```python
from build123d import *
from build123d.topology import SkipClean

# Parameters (mm, degrees)
SKETCH1_R           = 8.75
SKETCH1_R_2         = 4.25
SKETCH1_R_3         = 1.25
BOSS_EXTRUDE1_DEPTH = 1.8
SKETCH2_R           = 2
CUT_EXTRUDE1_DEPTH  = 0.6
SKETCH3_R           = 1.45
BOSS_EXTRUDE2_DEPTH = 1.5
FILLET1_R           = 5
CHAMFER1_SIZE       = 0.7
CHAMFER2_SIZE       = 0.7


with BuildPart() as part:
    # Sketch1 → Boss-Extrude1 (new body)
    with BuildSketch(Plane(origin=(0, 0, 0), x_dir=(1, 0, 0), z_dir=(0, 1, 0))):
        with Locations(Location((0, 0, 0), (0, 0, 270))):
            Circle(SKETCH1_R)
        with Locations(Location((0, 0, 0), (0, 0, 270))):
            Circle(SKETCH1_R_2, mode=Mode.SUBTRACT)
        with Locations(Location((-6, 0, 0), (0, 0, 270))):
            Circle(SKETCH1_R_3, mode=Mode.SUBTRACT)
        with Locations(Location((6, 0, 0), (0, 0, 270))):
            Circle(SKETCH1_R_3, mode=Mode.SUBTRACT)
    extrude(amount=BOSS_EXTRUDE1_DEPTH)

    # Sketch2 → Cut-Extrude1 (cut)
    with BuildSketch(Plane(origin=(0, 1.8, 0), x_dir=(1, 0, 0), z_dir=(0, 1, 0))):
        with Locations((-6, 0)):
            Circle(SKETCH2_R)
        with Locations((6, 0)):
            Circle(SKETCH2_R)
    extrude(amount=-CUT_EXTRUDE1_DEPTH, mode=Mode.SUBTRACT)

    # Sketch3 → Boss-Extrude2 (add)
    with SkipClean():  # the faces are left unmerged after this step: merging them gives an invalid solid
        with BuildSketch(Plane.XZ.offset(-1.8)):
            with BuildLine():
                Line((-22.592922776, -20.580461491), (-13.466151705, -20.580461491))
                ThreePointArc((-13.466151705, -20.580461491), (0, -11.838443279), (13.466151705, -20.580461491))
                Line((13.466151705, -20.580461491), (22.592922776, -20.580461491))
                Line((22.592922776, -20.580461491), (22.592922776, -12.644988276))
                ThreePointArc((22.592922776, -12.644988276), (15.601572689, 0), (22.592922776, 12.644988276))
                Line((22.592922776, 12.644988276), (22.592922776, 20.580461491))
                Line((22.592922776, 20.580461491), (13.466151705, 20.580461491))
                ThreePointArc((13.466151705, 20.580461491), (0, 11.838443279), (-13.466151705, 20.580461491))
                Line((-13.466151705, 20.580461491), (-22.592922776, 20.580461491))
                Line((-22.592922776, 20.580461491), (-22.592922776, 12.644988276))
                ThreePointArc((-22.592922776, 12.644988276), (-15.601572689, 0), (-22.592922776, -12.644988276))
                Line((-22.592922776, -12.644988276), (-22.592922776, -20.580461491))
            make_face()
            with Locations(Location((18.75, 16.75, 0), (0, 0, 270))):
                Circle(SKETCH3_R, mode=Mode.SUBTRACT)
            with Locations(Location((18.75, -16.75, 0), (0, 0, 270))):
                Circle(SKETCH3_R, mode=Mode.SUBTRACT)
            with Locations(Location((-18.75, -16.75, 0), (0, 0, 270))):
                Circle(SKETCH3_R, mode=Mode.SUBTRACT)
            with Locations(Location((-18.75, 16.75, 0), (0, 0, 270))):
                Circle(SKETCH3_R, mode=Mode.SUBTRACT)
            with BuildLine():
                ThreePointArc((-4.171875, -0.81114671), (0, -4.25), (4.171875, -0.81114671))
                ThreePointArc((4.171875, -0.81114671), (8, 0), (4.171875, 0.81114671))
                ThreePointArc((4.171875, 0.81114671), (0, 4.25), (-4.171875, 0.81114671))
                ThreePointArc((-4.171875, 0.81114671), (-8, 0), (-4.171875, -0.81114671))
            make_face(mode=Mode.SUBTRACT)
        extrude(amount=-BOSS_EXTRUDE2_DEPTH)

    # Fillet1
    fillet1_edges = [part.edges().sort_by_distance(p)[0] for p in [
        (13.466151705, 2.55, 20.580461491),
        (22.592922776, 2.55, 20.580461491),
        (22.592922776, 2.55, 12.644988276),
        (22.592922776, 2.55, -12.644988276),
        (22.592922776, 2.55, -20.580461491),
        (13.466151705, 2.55, -20.580461491),
        (-13.466151705, 2.55, -20.580461491),
        (-22.592922776, 2.55, -20.580461491),
        (-22.592922776, 2.55, -12.644988276),
        (-22.592922776, 2.55, 12.644988276),
        (-22.592922776, 2.55, 20.580461491),
        (-13.466151705, 2.55, 20.580461491),
    ]]
    fillet(fillet1_edges, radius=FILLET1_R)

    # Chamfer1
    # the kernel refuses this chamfer: 0.7 mm, written as the material it takes off along each edge
    with BuildSketch(Plane(origin=(0, 0, 0), x_dir=(0, 0, 1), z_dir=(-1, 0, 0))) as chamfer1_piece_1:
        Polygon((8.75, CHAMFER1_SIZE), (8.75 - CHAMFER1_SIZE, 0), (8.75, 0), align=None)
    revolve(axis=Axis((0, 0, 0), (0, 1, 0)), mode=Mode.SUBTRACT)
    with BuildSketch(Plane(origin=(0, 0, 0), x_dir=(0, 0, 1), z_dir=(-1, 0, 0))) as chamfer1_piece_2:
        Polygon((4.25 + CHAMFER1_SIZE, 0), (4.25, CHAMFER1_SIZE), (4.25, 0), align=None)
    revolve(axis=Axis((0, 0, 0), (0, 1, 0)), mode=Mode.SUBTRACT)

    # Chamfer2
    chamfer2_edges = [part.edges().sort_by_distance(p)[0] for p in [
        (15.601572689, 3.3, 0),
        (16.993372755, 3.3, 20.580461491),
        (22.592922776, 3.3, 15.369960777),
        (16.993372755, 3.3, -20.580461491),
        (0, 3.3, -11.838443279),
        (-16.993372755, 3.3, -20.580461491),
        (-22.592922776, 3.3, -15.369960777),
        (-15.601572689, 3.3, 0),
        (-22.592922776, 3.3, 15.369960777),
        (-16.993372755, 3.3, 20.580461491),
        (0, 3.3, 11.838443279),
        (14.041165239, 3.3, 19.992377481),
        (21.128456682, 3.3, 19.115995397),
        (22.133326206, 3.3, 13.065483774),
        (-21.128456682, 3.3, 19.115995397),
        (-14.041165239, 3.3, 19.992377481),
        (-22.133326206, 3.3, 13.065483774),
        (-22.133326206, 3.3, -13.065483774),
        (14.041165239, 3.3, -19.992377481),
        (-21.128456682, 3.3, -19.115995397),
        (-14.041165239, 3.3, -19.992377481),
        (21.128456682, 3.3, -19.115995397),
        (22.133326206, 3.3, -13.065483774),
        (22.592922776, 3.3, -15.369960777),
    ]]
    chamfer(chamfer2_edges, length=CHAMFER2_SIZE)


solid = part.part
```
Source: CAD feature listing. Evaluate the final solid. Frame: model axes, mm. A direction names the side the tool comes from. Round coordinates to 2 decimals unless told otherwise and drop trailing zeros. Write each loop counter-clockwise with the first axis right and the second up, starting at its lowest first coordinate (ties: lowest second). Pieces come first, ordered by that corner, then holes. Notation, with made-up numbers: M 81.5,28 L 114.5,28 A26 ccw 114.5,62 Z; hole C 62.25,37 d4. An arc over 180 degrees is marked long. Answer as a JSON object with one key per item and string values. Group by question number.
(1) Section query C-C on x = -18.75. State how many separate pieces and enclosed holes the cut face has, then the cut area to 3 significant figures.
(2) First-contact query: pin 1 (1.5 mm diameter, centred on x = 7.5, y = 1, fed in from -Z); pin 2 (8 mm diameter, centred on x = -17.5, z = 6.5, fed in from -Y); pin 3 (3 mm diameter, centred on x = 6, z = 0, fed in from -Y); pin 4 (3 mm diameter, centred on x = 6, z = 0, fed in from +Y). Flat tips, straight axial feed; report the tip coordinate or a pass-through.
(3) Ray query, line 1 (Z direction, x = -18.5, y = 2); line 2 (Y direction, x = 12, z = 5.5); line 3 (Z direction, x = 18, y = 2.95). Return the intervals inside material, ascending. Write a range as [from, to].
(4) Mould query, pull axis X, two halves, no side actions, for faces 5 (the cylindrical face through (21.167, 2.206, 19.077)), 6 (the cylindrical face through (-0.2, 2.19, -11.84)), 7 (the cylindrical face through (-22.146, 2.206, -13.093)). Classes: +X half, -X half, draft (parallel to the pull), parting line (faces both ways), or undercut.
(5) Section query A-A on x = 0. Output: boundary loops of the cut face in (y, z), then the cut area to 3 significant figures.
(6) Section query B-B on z = 0. Output: boundary loops of the cut face in (x, y), then the cut area to 3 significant figures.
(7) Reachability of faces 1 (the cylindrical face through (-5.324, 1.242, -6.944)), 2 (the cylindrical face through (-14.071, 2.206, 20.008)), 3 (the flat face through (7, 1.2, 1)), 4 (the cylindrical face through (14.011, 2.206, -19.976)) from +Z, -Z, +X, -X, +Y, -Y: full face, straight path, thin tool, end or side. Return the list, or none.
Computed values:
{
 "1": {"separate pieces": "4", "enclosed holes": "0", "area": "23.8 mm^2"},
 "2": {"pin 1": "z = -5.57", "pin 2": "y = 1.8", "pin 3": "y = 0", "pin 4": "y = 1.2"},
 "3": {"line 1": "[-20.5, -18.18], [-15.32, -8.84], [8.84, 15.32], [18.18, 20.5]", "line 2": "[1.8, 3.3]", "line 3": "[-20.21, -17.99], [-15.51, -8.74], [8.74, 15.51], [17.99, 20.21]"},
 "4": {"face 5": "+X half", "face 6": "undercut", "face 7": "-X half"},
 "5": {"outline": "M 0,-8.05 L 0.7,-8.75 L 1.8,-8.75 L 1.8,-11.84 L 2.6,-11.84 L 3.3,-11.14 L 3.3,-4.25 L 0.7,-4.25 L 0,-4.95 Z; M 0,4.95 L 0.7,4.25 L 3.3,4.25 L 3.3,11.14 L 2.6,11.84 L 1.8,11.84 L 1.8,8.75 L 0.7,8.75 L 0,8.05 Z", "area": "37.5 mm^2"},
 "6": {"outline": "M -15.6,1.8 L -8.75,1.8 L -8.75,0.7 L -8.05,0 L -7.25,0 L -7.25,1.2 L -8,1.2 L -8,3.3 L -14.9,3.3 L -15.6,2.6 Z; M -4.75,0.2 L -4.25,0.7 L -4.25,1.2 L -4.75,1.2 Z; M 4.25,0.7 L 4.75,0.2 L 4.75,1.2 L 4.25,1.2 Z; M 7.25,0 L 8.05,0 L 8.75,0.7 L 8.75,1.8 L 15.6,1.8 L 15.6,2.6 L 14.9,3.3 L 8,3.3 L 8,1.2 L 7.25,1.2 Z", "area": "27.1 mm^2"},
 "7": {"face 1": "-Y", "face 2": "+Z, +Y, -Y", "face 3": "+Y", "face 4": "-Z, +Y, -Y"}
}
